Check sheet for the modelled part. Datum: model origin and axes. Units: mm. A direction names the side the tool comes from. Round coordinates to 2 decimals unless told otherwise and drop trailing zeros. Order: outer loops, then holes, each group sorted by start corner. A loop starts at its lowest first (then second) coordinate and runs counter-clockwise, first axis right, second up. Notation, with made-up numbers: (-1.75, -30) -> (52.25, -30) arc R5 cw to (52.25, -25) -> close; hole circle Ø6 at (62.5, 86.5). An arc over 180 degrees is marked (long way). Use CSV: the item, a comma, the result in double quotes.
```python
from build123d import *

# Parameters (mm, degrees)
SKETCH_1_W          = 15
SKETCH_1_H          = 15
SKETCH_1_W_2        = 13
SKETCH_1_H_2        = 13
EXTRUDE_1_DEPTH     = 280
SKETCH_2_R          = 1.5
CUT_EXTRUDE_1_DEPTH = 260
SKETCH_3_R          = 4
CUT_EXTRUDE_2_DEPTH = 2
SKETCH_4_R          = 1.5
CUT_EXTRUDE_3_DEPTH = 281.501782526
SKETCH_5_R          = 4
CUT_EXTRUDE_4_DEPTH = 2


with BuildPart() as part:
    # 草图1 → 凸台-拉伸1 (new body)
    with BuildSketch(Plane(origin=(0, 0, 0), x_dir=(1, 0, 0), z_dir=(0, 1, 0))):
        Rectangle(SKETCH_1_W, SKETCH_1_H)
        Rectangle(SKETCH_1_W_2, SKETCH_1_H_2, mode=Mode.SUBTRACT)
    extrude(amount=EXTRUDE_1_DEPTH)

    # 草图2 → 切除-拉伸1 (cut)
    with BuildSketch(Plane.ZY.offset(7.5)):
        with Locations((0, 220)):
            Circle(SKETCH_2_R)
        with Locations((0, 60)):
            Circle(SKETCH_2_R)
    extrude(amount=-CUT_EXTRUDE_1_DEPTH, mode=Mode.SUBTRACT)

    # 草图3 → 切除-拉伸2 (cut)
    with BuildSketch(Plane(origin=(7.5, 0, 0), x_dir=(0, 0, -1), z_dir=(1, 0, 0))):
        with Locations((0, 60)):
            Circle(SKETCH_3_R)
        with Locations((0, 220)):
            Circle(SKETCH_3_R)
    extrude(amount=-CUT_EXTRUDE_2_DEPTH, mode=Mode.SUBTRACT)

    # 草图4 → 切除-拉伸3 (cut, through all)
    with BuildSketch(Plane(origin=(7.5, 0, 0), x_dir=(0, 0, -1), z_dir=(1, 0, 0))):
        with Locations((0, 250)):
            Circle(SKETCH_4_R)
        with Locations(Location((0, 30, 0), (0, 0, 180))):
            Circle(SKETCH_4_R)
    extrude(amount=-CUT_EXTRUDE_3_DEPTH, mode=Mode.SUBTRACT)

    # 草图5 → 切除-拉伸4 (cut)
    with BuildSketch(Plane.ZY.offset(7.5)):
        with Locations((0, 250)):
            Circle(SKETCH_5_R)
        with Locations((0, 30)):
            Circle(SKETCH_5_R)
    extrude(amount=-CUT_EXTRUDE_4_DEPTH, mode=Mode.SUBTRACT)


solid = part.part
```
Q1. Go/stop test with a flat-tipped pin: pin 1 (6.5 mm diameter, centred on y = 220, z = 0, fed in from +X). Record where the tip stops, or that it passes through.
Result sheet:
pin 1,"stops at x = -6.5"
Q2. Sectioned sample at B-B, the plane y = 188.5. Enter the section's corners in (x, z).
Result sheet:
outline,"(-7.5, -7.5) -> (7.5, -7.5) -> (7.5, 7.5) -> (-7.5, 7.5) -> close; hole (-6.5, -6.5) -> (6.5, -6.5) -> (6.5, 6.5) -> (-6.5, 6.5) -> close"
Q3. Mould release check, pull along X, two halves, no side actions. Record for faces 4 (the face through (-7.5, 138, 0)), 5 (the face through (0, 138, 6.5)), 6 (the face through (-7, 0, 0)): pulls with the +X half, pulls with the -X half, needs draft (parallel to the pull), parting line crosses it, or undercut.
Result sheet:
face 4,"pulls with the -X half"
face 5,"undercut"
face 6,"needs draft"
Q4. Sectioned sample at A-A, the plane x = -1. Enter the section's corners in (y, z), then the cut area to 3 significant figures.
Result sheet:
outline,"(0, -7.5) -> (280, -7.5) -> (280, -6.5) -> (0, -6.5) -> close; (0, 6.5) -> (280, 6.5) -> (280, 7.5) -> (0, 7.5) -> close"
area,"560 mm^2"
Q5. Access from +Z, -Z, +X, -X, +Y, -Y to the whole of each face (thin tool, end or side, straight path). Record for faces 1 (the face through (-7.007, 253.373, 2.15)), 2 (the face through (6.5, 138, 0)), 3 (the face through (7.007, 56.095, 0.867)).
Result sheet:
face 1,"-X"
face 2,"+Y, -Y"
face 3,"+X"
Q6. Scan lines: L1, parallel to Y at x = 7.2, z = 0; L2, parallel to X at y = 56, z = 3.25; L3, parallel to Z at x = -7.05, y = 220. Record each from-to range of solid material in increasing order.
Result sheet:
L1,"y = 0 to 28.5, 31.5 to 56, 64 to 216, 224 to 248.5, 251.5 to 280"
L2,"x = -7.5 to -6.5, 6.5 to 7.5"
L3,"z = -7.5 to -1.5, 1.5 to 7.5"
